```python
from build123d import *

# Parameters (mm, degrees)
PAD_DEPTH    = 11
CHAMFER_SIZE = 3.1
FILLET_R     = 2
FILLET001_R  = 5


with BuildPart() as part:
    # Sketch → Pad (new body)
    with BuildSketch(Plane.XY):
        Polygon((-50.544724, -24.61614), (-50.544724, -29.61614), (-10.544724, -29.61614), (-10.544724, 20.38386), (39.455276, 20.38386), (39.455276, 25.38386), (-20.544724, 25.38386), (-20.544724, -24.61614), align=None)
    extrude(amount=PAD_DEPTH)

    # Chamfer
    chamfer_edges = [part.edges().sort_by_distance(p)[0] for p in [
        (-30.544724, -29.61614, 0),
        (-30.544724, -29.61614, 11),
    ]]
    chamfer(chamfer_edges, length=CHAMFER_SIZE)

    # Fillet
    fillet_edges = [part.edges().sort_by_distance(p)[0] for p in [
        (39.455276, 25.38386, 5.5),
        (-20.544724, 25.38386, 5.5),
    ]]
    fillet(fillet_edges, radius=FILLET_R)

    # Fillet001
    fillet001_edges = [part.edges().sort_by_distance(p)[0] for p in [
        (-10.544724, 20.38386, 5.5),
    ]]
    fillet(fillet001_edges, radius=FILLET001_R)


solid = part.part
```
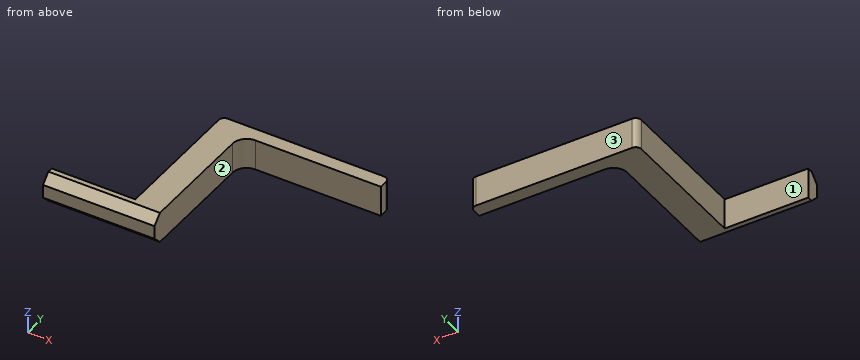
Build history of the part. All positions in model axes, mm. Face numbers are marked on the shaded views. A direction names the side the tool comes from. Round coordinates to 2 decimals unless told otherwise and drop trailing zeros. Order: outer loops, then holes, each group sorted by start corner. A loop starts at its lowest first (then second) coordinate and runs counter-clockwise, first axis right, second up. Notation, with made-up numbers: (28, 64.5) -> (51, 64.5) arc R33 cw to (51, 99.5) -> close; hole circle Ø5 at (80, 26). An arc over 180 degrees is marked (long way). Answer in a Markdown table with one row per item.
1) Band-saw the part on A-A on z = 6.25. Give the cut face in (x, y), and give its area (3 significant figures).
Values:
| item | result |
|---|---|
| outline | (-50.54, -29.62) -> (-10.54, -29.62) -> (-10.54, 15.38) arc R5 cw to (-5.54, 20.38) -> (39.46, 20.38) -> (39.46, 23.38) arc R2 ccw to (37.46, 25.38) -> (-18.54, 25.38) arc R2 ccw to (-20.54, 23.38) -> (-20.54, -24.62) -> (-50.54, -24.62) -> close |
| area | 954 mm2 |
2) Pin check, flat tips, straight feed: P1, Ø1, axis at x = 19, z = 3, coming from the -Y side; P2, Ø1.5, axis at y = 17.5, z = 6, coming from the -X side; P3, Ø5.5, axis at x = -38.5, z = 8, coming from the +Y side. Stop position of each tip, or through.
Values:
| item | result |
|---|---|
| P1 | y = 20.38 |
| P2 | x = -20.54 |
| P3 | y = -24.62 |
3) Band-saw the part on C-C on y = 8.5. Give the cut face in (x, z).
Values:
| item | result |
|---|---|
| outline | (-20.54, 0) -> (-10.54, 0) -> (-10.54, 11) -> (-20.54, 11) -> close |
4) Which spindle directions (+Z, -Z, +X, -X, +Y, -Y) get a long thin tool onto all of the face, cutting with end or side? Do the marked faces 1, 2 and 3. Say none if no direction does.
Values:
| item | result |
|---|---|
| face 1 | +Z, -Z, -X, +Y |
| face 2 | +Z, -Z, +X, -Y |
| face 3 | +Z, -Z, +X, -X, +Y |
5) Band-saw the part on B-B on x = -36.5. Give the cut face in (y, z), and give its area (3 significant figures).
Values:
| item | result |
|---|---|
| outline | (-29.62, 3.1) -> (-26.52, 0) -> (-24.62, 0) -> (-24.62, 11) -> (-26.52, 11) -> (-29.62, 7.9) -> close |
| area | 45.4 mm2 |
6) Wall check: L1, parallel to Y at x = -5.5, z = 5; L2, parallel to X at y = -12, z = 2; L3, parallel to Y at x = -27, z = 7.5. Give the ranges that are in metal, low to high.
Values:
| item | result |
|---|---|
| L1 | 20.38 to 25.38 |
| L2 | -20.54 to -10.54 |
| L3 | -29.62 to -24.62 |
7) Band-saw the part on D-D on z = 1.25. Give the cut face in (x, y), and give its area (3 significant figures).
Values:
| item | result |
|---|---|
| outline | (-50.54, -27.77) -> (-10.54, -27.77) -> (-10.54, 15.38) arc R5 cw to (-5.54, 20.38) -> (39.46, 20.38) -> (39.46, 23.38) arc R2 ccw to (37.46, 25.38) -> (-18.54, 25.38) arc R2 ccw to (-20.54, 23.38) -> (-20.54, -24.62) -> (-50.54, -24.62) -> close |
| area | 880 mm2 |
